For this review, use the dimensioned drawing (mm, ordinates from the lowest corner) and the shaded views. A direction names the side the tool comes from. Give positions to 0.01 mm unless a question says otherwise; leave off trailing zeros. Write each loop counter-clockwise with the first axis right and the second up, starting at its lowest first coordinate (ties: lowest second). Pieces come first, ordered by that corner, then holes.
1) Machinability: for the marked faces 1 and 2, which of the approach directions +Z, -Z, +X, -X, +Y, -Y give a long, thin tool a straight path to every point of the face, cutting with its end or side? Answer none if there is none.
2) Wall thickness on line 1 along X through (y, z) = (56, 5) (1 decimal); line 2 along Y through (x, z) = (48.5, 28) (1 decimal); line 3 along X through (y, z) = (55, 29) (1 decimal): over which ranges is each line inside the solid? List them lowest first.
3) For P1, Ø10, axis at y = 24.5, z = 15.5, coming from the -X side; P2, Ø12, axis at y = 53.5, z = 17, coming from the -X side; P3, Ø4, axis at x = 29, z = 28.5, coming from the -Y side, all flat-tipped, find the tip position at first contact; note any pin that passes through.
4) We need section C-C on z = 15.5. Give the boundary of the cut face in (x, y).
5) Draft analysis for pull direction Y (two halves, no side actions). For the marked faces 3 and 4, state which applies: pulls with the +Y half, pulls with the -Y half, needs draft (parallel to the pull), parting line crosses it, or undercut.
6) We need section D-D on y = 24. Give the boundary of the cut face in (x, z).
7) We need section A-A on x = 36.25. Give the boundary of the cut face in (y, z).
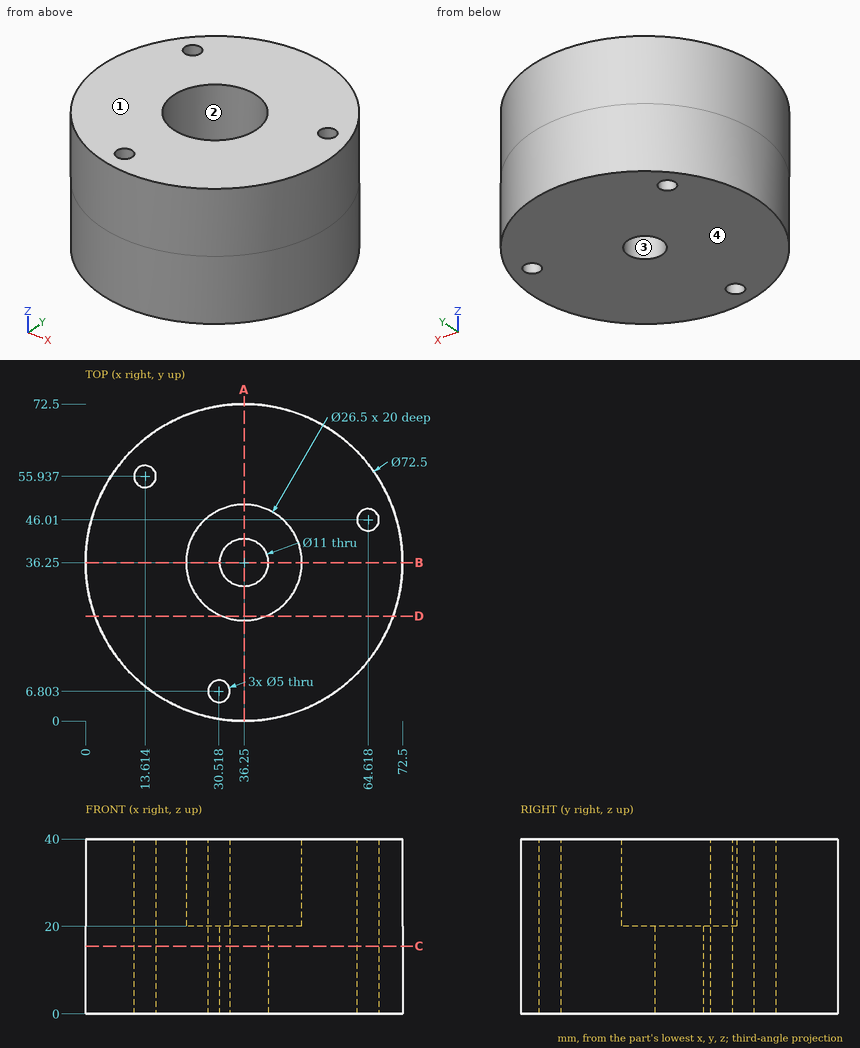
Results list:
1. face 1: +Z, +X, -X, +Y, -Y
1. face 2: +Z
2. line 1: x = 5.9 to 11.1, 16.1 to 66.6
2. line 2: y = 2.1 to 31.2, 41.3 to 70.4
2. line 3: x = 5.2 to 11.3, 15.9 to 67.3
3. P1: stops at x = 0.63
3. P2: stops at x = 1.79
3. P3: stops at y = 0.38
4. outline: circle Ø72.5 at (36.25, 36.25); hole circle Ø5 at (13.61, 55.94); hole circle Ø5 at (30.52, 6.8); hole circle Ø11 at (36.25, 36.25); hole circle Ø5 at (64.62, 46.01)
5. face 3: undercut
5. face 4: needs draft
6. outline: (2.13, 0) - (70.37, 0) - (70.37, 40) - (41.3, 40) - (41.3, 20) - (31.2, 20) - (31.2, 40) - (2.13, 40) - close
7. outline: (0, 0) - (30.75, 0) - (30.75, 20) - (23, 20) - (23, 40) - (0, 40) - close; (41.75, 0) - (72.5, 0) - (72.5, 40) - (49.5, 40) - (49.5, 20) - (41.75, 20) - close
